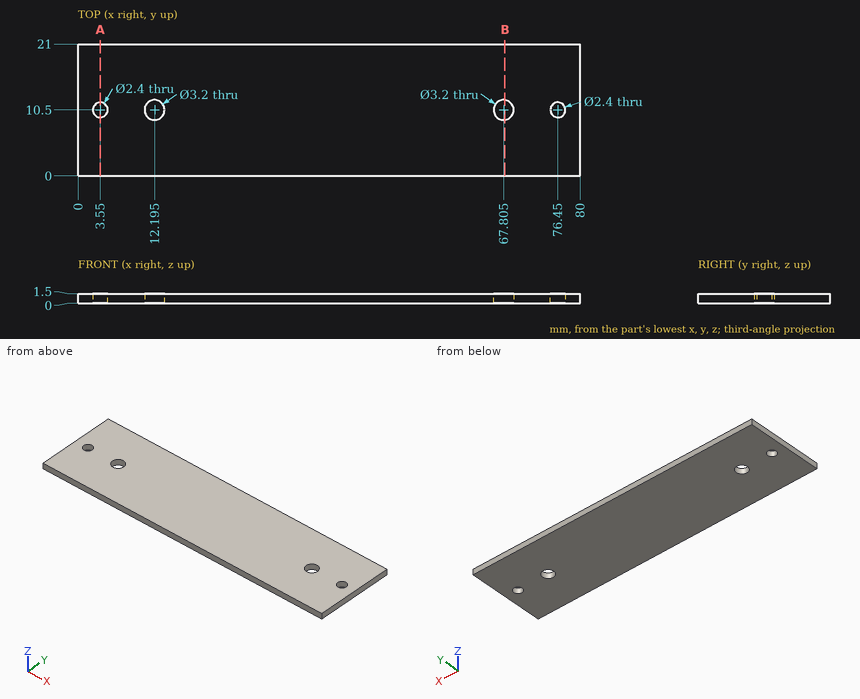
Job drawing, mm, ordinate dimensions from the low corner. One solid piece. Round coordinates to 2 decimals unless told otherwise and drop trailing zeros. Loops run counter-clockwise (first coordinate to the right, second up) from the corner with the lowest first, then second, coordinate; pieces in that order, holes last. Notation, with made-up numbers: M -10.75,48.5 L 37.25,48.5 A24 cw 37.25,78.5 Z; hole C 1.25,-10 d2. An arc over 180 degrees is marked long. One line per question, with ' | ' between items. Start each with the question number.
Item 1: Cut at B-B, the plane x = 68. Write the cut outline in (y, z), plus the area to 3 significant figures.
Item 2: Wall check: line 1 (X direction, y = 9.25, z = 0.1); line 2 (Y direction, x = 76.45, z = 0.45); line 3 (Y direction, x = 76, z = 0.9). Give the ranges that are in metal, low to high.
Item 3: Cut at A-A, the plane x = 3.55. Write the cut outline in (y, z).
Responses:
1) outline: M 0,0 L 8.91,0 L 8.91,1.5 L 0,1.5 Z; M 12.09,0 L 21,0 L 21,1.5 L 12.09,1.5 Z | area: 26.7 mm²
2) line 1: x = 0 to 11.2, 13.19 to 66.81, 68.8 to 80 | line 2: y = 0 to 9.3, 11.7 to 21 | line 3: y = 0 to 9.39, 11.61 to 21
3) outline: M 0,0 L 9.3,0 L 9.3,1.5 L 0,1.5 Z; M 11.7,0 L 21,0 L 21,1.5 L 11.7,1.5 Z
